The listing builds one solid part. Answer for the finished solid, in the listing's coordinates (mm). A direction names the side the tool comes from. Round coordinates to 2 decimals unless told otherwise and drop trailing zeros. Write each loop counter-clockwise with the first axis right and the second up, starting at its lowest first coordinate (ties: lowest second). Pieces come first, ordered by that corner, then holes. Notation, with made-up numbers: (78, 5) - (96, 5) arc R19 ccw to (96, 15) - close; hole circle Ø1 at (82, 61). An arc over 180 degrees is marked (long way). Answer in a Markdown table with one row per item.
Autodesk Inventor part; units mm, degrees
ref_plane "Plano de trabajo1" through (0, 0, -565.5) normal (0, 0, 1) x (1, 0, 0)
ref_plane "YZ Plane" through (0, 0, 0) normal (1, 0, 0) x (0, 1, 0)
ref_plane "XZ Plane" through (0, 0, 0) normal (0, 1, 0) x (-1, 0, 0)
sketch "Boceto1" plane through (0, 0, 0) normal (0, 0, 1) x (1, 0, 0)
  line L0 (28.1307, 40.0149) -> (1.9307, 40.0149)
  line L1 (1.9307, 41.4149) -> (28.1307, 41.4149)
  line L2 (0.0307, -0.1851) -> (0.0307, 51.6749)
  line L3 (24.8307, 55.8149) -> (24.8307, 54.1749)
  line L4 (28.6307, 54.4149) -> (28.6307, 47.9149)
  line L5 (28.6307, 46.5149) -> (24.8307, 46.5149)
  line L6 (24.8307, 46.5149) -> (24.8307, 48.1549)
  line L7 (26.2307, 47.9149) -> (28.6307, 47.9149)
  line L8 (26.2307, 49.1649) -> (25.5249, 49.1649)
  line L9 (25.5249, 49.1649) -> (24.8307, 48.1549)
  line L10 (26.2307, 53.1649) -> (25.5249, 53.1649)
  line L11 (1.4307, 41.9149) -> (1.4307, 48.9149)
  line L12 (1.4307, 48.9149) -> (2.9307, 48.9149)
  line L13 (2.9307, 48.9149) -> (2.9307, 51.6749)
  line L14 (4.1707, 55.8149) -> (10.8307, 55.8149)
  line L15 (9.3926, 54.4149) -> (5.6707, 54.4149)
  line L16 (10.8307, 55.8149) -> (10.8307, 53.3149)
  line L17 (10.8307, 53.3149) -> (10.1207, 53.3149)
  line L18 (10.1207, 53.3149) -> (9.3926, 54.4149)
  line L19 (26.2307, 54.4149) -> (28.6307, 54.4149)
  arc A0 (5.6707, 54.4149) -> (2.9307, 51.6749) centre (5.6707, 51.6749) ccw
  arc A1 (4.1707, 55.8149) -> (0.0307, 51.6749) centre (4.1707, 51.6749) ccw
  line L20 (24.8307, 54.1749) -> (25.5249, 53.1649)
  line L21 (26.2307, 54.4149) -> (26.2307, 53.1649)
  line L22 (26.2307, 47.9149) -> (26.2307, 49.1649)
  arc A2 (1.9307, 40.0149) -> (1.4307, 39.5149) centre (1.9307, 39.5149) ccw
  arc A3 (28.6307, 39.5149) -> (28.1307, 40.0149) centre (28.1307, 39.5149) ccw
  arc A4 (28.1307, 41.4149) -> (28.6307, 41.9149) centre (28.1307, 41.9149) ccw
  arc A5 (1.4307, 41.9149) -> (1.9307, 41.4149) centre (1.9307, 41.9149) ccw
  line L23 (30.0307, 55.8149) -> (24.8307, 55.8149)
  line L24 (28.6307, 41.9149) -> (28.6307, 46.5149)
  line L25 (30.0307, 55.8149) -> (30.0307, -0.1851)
  line L26 (1.4307, 29.0149) -> (28.6307, 29.0149)
  line L27 (1.4307, 27.6149) -> (28.6307, 27.6149)
  line L28 (1.4307, 39.5149) -> (1.4307, 29.0149)
  line L29 (1.4307, 27.6149) -> (1.4307, 1.2149)
  line L30 (28.6307, 1.2149) -> (28.6307, 27.6149)
  line L31 (28.6307, 29.0149) -> (28.6307, 39.5149)
  line L32 (28.6307, 39.5149) -> (28.6307, 29.0149)
  line L33 (28.6307, 27.6149) -> (28.6307, 1.2149)
  line L34 (4.5307, 5.9149) -> (6.8307, 5.9149)
  line L35 (7.8307, 4.9149) -> (7.8307, 2.5149)
  line L36 (7.8307, 2.5149) -> (6.4307, 2.5149)
  line L37 (6.4307, 2.5149) -> (6.4307, 4.5149)
  line L38 (6.4307, 4.5149) -> (4.9307, 4.5149)
  line L39 (4.9307, 4.5149) -> (4.9307, -3.4851)
  line L40 (4.9307, -3.4851) -> (6.4307, -3.4851)
  line L41 (6.4307, -3.4851) -> (6.4307, -1.4851)
  line L42 (6.4307, -1.4851) -> (7.8307, -1.4851)
  line L43 (7.8307, -1.4851) -> (7.8307, -3.8851)
  line L44 (6.8307, -4.8851) -> (3.5307, -4.8851)
  line L45 (3.5307, -4.8851) -> (3.5307, -0.1851)
  arc A6 (7.8307, 4.9149) -> (6.8307, 5.9149) centre (6.8307, 4.9149) ccw
  arc A7 (4.5307, 5.9149) -> (3.5307, 4.9149) centre (4.5307, 4.9149) ccw
  arc A8 (6.8307, -4.8851) -> (7.8307, -3.8851) centre (6.8307, -3.8851) ccw
  line L46 (3.5307, 1.2149) -> (1.4307, 1.2149)
  line L47 (3.5307, -0.1851) -> (0.0307, -0.1851)
  line L48 (3.5307, 1.2149) -> (3.5307, 4.9149)
  line L49 (25.5307, 5.9149) -> (23.2307, 5.9149)
  line L50 (22.2307, 4.9149) -> (22.2307, 2.5149)
  line L51 (22.2307, 2.5149) -> (23.6307, 2.5149)
  line L52 (23.6307, 2.5149) -> (23.6307, 4.5149)
  line L53 (23.6307, 4.5149) -> (25.1307, 4.5149)
  line L54 (25.1307, 4.5149) -> (25.1307, -3.4851)
  line L55 (25.1307, -3.4851) -> (23.6307, -3.4851)
  line L56 (23.6307, -3.4851) -> (23.6307, -1.4851)
  line L57 (23.6307, -1.4851) -> (22.2307, -1.4851)
  line L58 (22.2307, -1.4851) -> (22.2307, -3.8851)
  line L59 (23.2307, -4.8851) -> (26.5307, -4.8851)
  line L60 (26.5307, -4.8851) -> (26.5307, -0.1851)
  arc A9 (23.2307, 5.9149) -> (22.2307, 4.9149) centre (23.2307, 4.9149) ccw
  arc A10 (26.5307, 4.9149) -> (25.5307, 5.9149) centre (25.5307, 4.9149) ccw
  arc A11 (22.2307, -3.8851) -> (23.2307, -4.8851) centre (23.2307, -3.8851) ccw
  line L61 (26.5307, 1.2149) -> (28.6307, 1.2149)
  line L62 (26.5307, -0.1851) -> (30.0307, -0.1851)
  line L63 (26.5307, 1.2149) -> (26.5307, 4.9149)
  point P0 (28.6307, 51.1649)
  point P1 (0.0307, 0.7149)
  point P2 (4.9307, 0.5149)
  point P3 (25.1307, 0.5149)
  dimension "d31" = 1.4
  dimension "d42" = 2.5
  dimension "d43" = 0.71
  dimension "d45" = 2.9
  dimension "d47" = 33.5
  dimension "d48" = 7.5
  dimension "d51" = 2.74
  dimension "d59" = 6.9
  dimension "d60" = 1.4
  dimension "d78" = 6.5
  dimension "d84" = 1.4
  dimension "d85" = 1.4
  dimension "d88" = 2.4
  dimension "d95" = 6.02
  dimension "d99" = 111
  dimension "d100" = 2.4
  dimension "d108" = 4
  dimension "d109" = 0.7058
  dimension "d110" = 0.7058
  dimension "d143" = 1.4
  dimension "d147" = 1.4
  dimension "d148" = 30
  dimension "d149" = 1.4
  dimension "d150" = 14
  dimension "d151" = 27.2
  dimension "d152" = 14.4
  dimension "d153" = 1.4
  dimension "d154" = 11
  dimension "d155" = 1.4
  dimension "d156" = 1.4
  dimension "d157" = 1.4
  dimension "d158" = 1.4
  dimension "d162" = 60.7
  dimension "d163" = 10.8
  dimension "d164" = 8
  dimension "d165" = 2
  dimension "d166" = 4
  dimension "d167" = 1.5
  dimension "d168" = 7.8
  dimension "d169" = 1
  dimension "d172" = 1.4
  dimension "d173" = 4.7
  dimension "d175" = 56
  dimension "d176" = 13.8
  dimension "d177" = 14.4
  dimension "d180" = 1.5
  dimension "d181" = 4.14
  dimension "d182" = 10.8
  dimension "d183" = 14.4
  dimension "d184" = 0.5
  dimension "d187" = 3.5
  dimension "d188" = 4.9
  dimension "d189" = 6.4
  dimension "d190" = 7.8
  dimension "d191" = 26.5
  dimension "d193" = 54.6
  dimension "d195" = 3.5
  dimension "d196" = 4.9
  dimension "d197" = 53.9
  dimension "d198" = 53.7
  dimension "d202" = 2
  dimension "d203" = 3.01
  dimension "d204" = 2
  dimension "d205" = 9.3
extrude "Extrusión1" add sketch "Boceto1" against normal blind 1131
ref_plane "Plano de trabajo1" through (0, 0, -565.5) normal (0, 0, 1) x (1, 0, 0)
sketch "Boceto2" plane through (30.0307, -0.1851, 0) normal (1, 0, 0) x (0, 0, -1)
  line L0 (0, -4.7) -> (0, 0)
  line L1 (0, -4.7) -> (1131, -4.7)
  line L2 (1131, 0) -> (1131, -4.7)
  line L3 (0, 0) -> (1131, 0)
  line L4 (0, 0) -> (0, 56)
  line L5 (0, 0) -> (1131, 0)
  line L6 (1131, 56) -> (1131, 0)
  line L7 (0, 56) -> (1131, 56)
  line L8 (0, -4.7) -> (60.7, 56)
  line L9 (0, 56) -> (60.7, 56)
  line L10 (0, 56) -> (0, -4.7)
  point P0 (0, 0.1851)
  point P1 (0, 0)
  dimension "d201" = 45
extrude "Extrusión2" cut sketch "Boceto2" against normal through all contours L0 L3 L8 | L4 L7 L8 L3
mirror "Simetría1" about plane through (0, 0, -565.5) normal (0, 0, 1) of "Extrusión2"
ref_plane "Plano de trabajo2" through (15.0307, -0.1851, -1126.3) normal (-1, 0, 0) x (0, 0, 1)
properties part number "SP40-10 HOJA CORREDERA 1131 mm" material "Aluminio"
(1) Section A-A (x = 17) is taken. Give the vertices of the cut face in (y, z).
Checked values:
| item | result |
|---|---|
| outline | (27.61, -1098.5) - (29.01, -1097.1) - (29.01, -33.9) - (27.61, -32.5) - close; (40.01, -1086.1) - (41.41, -1084.7) - (41.41, -46.3) - (40.01, -44.9) - close |
(2) Flat-ended cylindrical pins translate along their axes: pin 1 (2 mm diameter, centred on x = 11.5, z = -376.5, fed in from -Y); pin 2 (12 mm diameter, centred on x = 4, y = 45, fed in from -Z); pin 3 (1 mm diameter, centred on x = 28, z = -668.5, fed in from -Y). Find the tip coordinate at first contact, or state that the pin passes through.
Checked values:
| item | result |
|---|---|
| pin 1 | stops at y = 27.61 |
| pin 2 | stops at z = -1086.54 |
| pin 3 | stops at y = -0.19 |
(3) For faces 5 (the flat face through (15, 27.615, -558)), 6 (the flat face through (13.99, 27.855, -1098.26)), determine the directions among +Z, -Z, +X, -X, +Y, -Y from which every point of the face is accessible in a straight line to the end or side of a thin tool.
Checked values:
| item | result |
|---|---|
| face 5 | +Z, -Z |
| face 6 | -Z, +X, -X, +Y |
(4) Find the intervals of material crossed by line 1 (X direction, y = 1.5, z = -1075); line 2 (Y direction, x = 7.25, z = -562.5); line 3 (Y direction, x = 22.5, z = -596.5), in increasing order.
Checked values:
| item | result |
|---|---|
| line 1 | x = 0.03 to 1.43, 3.53 to 4.93, 25.13 to 26.53, 28.63 to 30.03 |
| line 2 | y = -4.79 to -1.49, 2.51 to 5.82, 27.61 to 29.01, 40.01 to 41.41, 54.41 to 55.81 |
| line 3 | y = -4.57 to -1.49, 2.51 to 5.6, 27.61 to 29.01, 40.01 to 41.41 |
(5) For a pull along X with two mould halves and no side action, classify faces 1 (the flat face through (30.031, 28, -558)), 2 (the flat face through (15, 40.015, -558)), 3 (the flat face through (28.631, 14, -558)), 4 (the flat face through (0.031, 25, -558)) as pulls with the +X half, pulls with the -X half, needs draft (parallel to the pull), parting line crosses it, or undercut.
Checked values:
| item | result |
|---|---|
| face 1 | pulls with the +X half |
| face 2 | undercut |
| face 3 | undercut |
| face 4 | pulls with the -X half |
